```python
from build123d import *

# Parameters (mm, degrees)
SKETCH_1_R          = 1.6
SKETCH_1_R_2        = 2.1
EXTRUDE_1_DEPTH     = 6
CUT_EXTRUDE_1_DEPTH = 10
FILLET_1_R          = 3
FILLET_2_R          = 3


with BuildPart() as part:
    # 草图1 → 凸台-拉伸1 (new body)
    with BuildSketch(Plane(origin=(0, 0, 0), x_dir=(0, 0, -1), z_dir=(1, 0, 0))):
        Polygon((285, 10), (-28.22, 10), (-28.22, -34), (115, -34), (165, -10), (285, -10), align=None)
        Circle(SKETCH_1_R, mode=Mode.SUBTRACT)
        with Locations((135, 0)):
            Circle(SKETCH_1_R, mode=Mode.SUBTRACT)
        with Locations((270, 0)):
            Circle(SKETCH_1_R, mode=Mode.SUBTRACT)
        with Locations((97.86, -27)):
            Circle(SKETCH_1_R_2, mode=Mode.SUBTRACT)
        with Locations((97.86, -19)):
            Circle(SKETCH_1_R_2, mode=Mode.SUBTRACT)
        with Locations((97.86, -11)):
            Circle(SKETCH_1_R_2, mode=Mode.SUBTRACT)
        with Locations((97.86, -3)):
            Circle(SKETCH_1_R_2, mode=Mode.SUBTRACT)
        with Locations((97.86, 5)):
            Circle(SKETCH_1_R_2, mode=Mode.SUBTRACT)
        with Locations((-20.23, -27)):
            Circle(SKETCH_1_R_2, mode=Mode.SUBTRACT)
        with Locations((-20.23, -19)):
            Circle(SKETCH_1_R_2, mode=Mode.SUBTRACT)
        with Locations((-20.23, -11)):
            Circle(SKETCH_1_R_2, mode=Mode.SUBTRACT)
        with Locations((-20.23, -3)):
            Circle(SKETCH_1_R_2, mode=Mode.SUBTRACT)
        with Locations((-20.23, 5)):
            Circle(SKETCH_1_R_2, mode=Mode.SUBTRACT)
    extrude(amount=EXTRUDE_1_DEPTH)

    # 草图2 → 切除-拉伸1 (cut)
    with BuildSketch(Plane(origin=(6, 0, 0), x_dir=(0, 0, -1), z_dir=(1, 0, 0))):
        Polygon((13.2925, -0.009366832), (-9.032216719, -28), (35.617216719, -28), align=None)
        with BuildLine():
            ThreePointArc((3.290130805, -4.531560359), (1.729633197, -5.326196486), (0, -5.6))
            Line((0, -5.6), (-12.23, -5.6))
            Line((-12.23, -5.6), (-12.23, -23.990633168))
            Line((-12.23, -23.990633168), (3.290130805, -4.531560359))
        make_face()
        Polygon((61.139716719, 4), (16.490283281, 4), (38.815, -23.990633168), align=None)
        Polygon((64.3375, -0.009366832), (42.012783281, -28), (86.662216719, -28), align=None)
        Polygon((89.86, 4), (67.535283281, 4), (89.86, -23.990633168), align=None)
        Polygon((126.119901445, -23.116277457), (105.86, 1.103590865), (105.86, -29), (113.862146147, -29), align=None)
        Polygon((128.44547948, 5), (109.11934328, 5), (128.44547948, -18.103590865), align=None)
        Polygon((133.44547948, -19.6), (153.44547948, -10), (133.44547948, -10), align=None)
        with BuildLine():
            Line((152.5, -5), (172.5, -5))
            ThreePointArc((172.5, -5), (177.5, 0), (172.5, 5))
            Line((172.5, 5), (152.5, 5))
            ThreePointArc((152.5, 5), (147.5, 0), (152.5, -5))
        make_face()
        with BuildLine():
            Line((192.5, -5), (212.5, -5))
            ThreePointArc((212.5, -5), (217.5, 0), (212.5, 5))
            Line((212.5, 5), (192.5, 5))
            ThreePointArc((192.5, 5), (187.5, 0), (192.5, -5))
        make_face()
        with BuildLine():
            Line((232.5, -5), (252.5, -5))
            ThreePointArc((252.5, -5), (257.5, 0), (252.5, 5))
            Line((252.5, 5), (232.5, 5))
            ThreePointArc((232.5, 5), (227.5, 0), (232.5, -5))
        make_face()
    extrude(amount=-CUT_EXTRUDE_1_DEPTH, mode=Mode.SUBTRACT)

    # 圆角1
    fillet_1_edges = [part.edges().sort_by_distance(p)[0] for p in [
        (3, -23.116277457, -126.119901445),
        (3, -29, -113.862146147),
        (3, -29, -105.86),
        (3, 1.103590865, -105.86),
        (3, -18.103590865, -128.44547948),
        (3, 5, -109.11934328),
        (3, 5, -128.44547948),
        (3, 4, -61.139716719),
        (3, -23.990633168, -38.815),
        (3, -28, -86.662216719),
        (3, -28, -42.012783281),
        (3, -0.009366832, -64.3375),
        (3, -28, -35.617216719),
        (3, -28, 9.032216719),
        (3, -0.009366832, -13.2925),
        (3, 4, -89.86),
        (3, -23.990633168, -89.86),
        (3, 4, -67.535283281),
        (3, -4.531560359, -3.290130805),
        (3, -23.990633168, 12.23),
        (3, -5.6, 12.23),
        (3, -10, -133.44547948),
        (3, -10, -153.44547948),
        (3, -19.6, -133.44547948),
        (3, 4, -16.490283281),
    ]]
    fillet(fillet_1_edges, radius=FILLET_1_R)

    # 圆角2
    fillet_2_edges = [part.edges().sort_by_distance(p)[0] for p in [
        (3, -10, -285),
        (3, -10, -165),
        (3, -34, -115),
        (3, -34, 28.22),
        (3, 10, 28.22),
        (3, 10, -285),
    ]]
    fillet(fillet_2_edges, radius=FILLET_2_R)


solid = part.part
```
Input: part model. Units: mm. Frame: model coordinates. Coordinates: 2 decimals unless noted, no trailing zeros. Write each loop counter-clockwise with the first axis right and the second up, starting at its lowest first coordinate (ties: lowest second). Pieces come first, ordered by that corner, then holes. Notation, with made-up numbers: M 1.5,79 L 58.5,79 A31 ccw 58.5,117 Z; hole C 63.5,7 d4. An arc over 180 degrees is marked long. Use one line per item in the form item = value.
Q1. First-contact query: pin 1 (1.5 mm diameter, centred on x = 4.5, y = -13.5, fed in from -Z); pin 2 (2.5 mm diameter, centred on y = 0, z = -270, fed in from +X); pin 3 (1.8 mm diameter, centred on x = 3, z = -121, fed in from -Y). Flat tips, straight axial feed; report the tip coordinate or a pass-through.
Answer below:
pin_1 = -159.27
pin_2 = through
pin_3 = -31.55
Q2. Material intervals for probe 1 along Y at (x, z) = (3.7, 20.23); probe 2 along Y at (x, z) = (5.25, -121); probe 3 along Y at (x, z) = (3.5, -70), sorted ascending. Write a range as from..to.
Answer below:
probe_1 = -34..-29.1, -24.9..-21.1, -16.9..-13.1, -8.9..-5.1, -0.9..2.9, 7.1..10
probe_2 = -31.12..-25.57, -17..-9.2, 5..10
probe_3 = -34..-28, -7.11..10
Q3. Draft query along Y for faces 1 (the face through (3, 10, -131)), 2 (the face through (2.96, 2.34, -71.08)), 3 (the face through (3, -34, -44)). Return one class per face: released by +Y, released by -Y, zero draft, split by the parting line, or undercut.
Answer below:
face_1 = released by +Y
face_2 = undercut
face_3 = released by -Y
Q4. Section C-C (z = -263). Return loops of the section in (x, y).
Answer below:
outline = M 0,-10 L 6,-10 L 6,10 L 0,10 Z
Q5. Section A-A (z = -51). Return loops of the section in (x, y).
Answer below:
outline = M 0,-34 L 6,-34 L 6,-28 L 0,-28 Z; M 0,-16.73 L 6,-16.73 L 6,-8.71 L 0,-8.71 Z; M 0,4 L 6,4 L 6,10 L 0,10 Z
Q6. Section B-B (x = 1.75). Count the separate pieces of the cut face and the enclosed holes in it, plus the area to 3 significant figures.
Answer below:
separate_pieces = 1
enclosed_holes = 24
area = 6,520 mm²
